from build123d import *

# Parameters (mm, degrees)
F1_DEPTH = 2.54
F3_DEPTH = 22.86
F5_DEPTH = 38.1
F6_R     = 1.5875
F7_DEPTH = 254


with BuildPart() as f1:
    # F0 (on Top) → F1 (new body)
    with BuildSketch(Plane.XY):
        with BuildLine():
            Line((-152.4, 0), (0, 0))
            Line((0, 0), (0, 85.725))
            ThreePointArc((0, 85.725), (-76.2, 9.525), (-152.4, 85.725))
            Line((-152.4, 85.725), (-152.4, 0))
        make_face()
        with BuildLine():
            ThreePointArc((-152.4, 85.725), (-76.2, 9.525), (0, 85.725))
            Line((0, 85.725), (-152.4, 85.725))
        make_face()
        with BuildLine():
            Line((-152.4, 85.725), (0, 85.725))
            ThreePointArc((0, 85.725), (-76.2, 161.925), (-152.4, 85.725))
        make_face()
    extrude(amount=F1_DEPTH)

    # F2 (on face) → F3 (join)
    with BuildSketch(Plane.XY.offset(2.54)):
        with BuildLine():
            Line((-152.4, 85.725), (0, 85.725))
            ThreePointArc((0, 85.725), (-76.2, 161.925), (-152.4, 85.725))
        make_face()
    extrude(amount=F3_DEPTH)

    # F4 (on face) → F5 (join)
    with BuildSketch(Plane.XY.offset(2.54)):
        Polygon((-3.81, 3.81), (-148.59, 3.81), (-148.59, 85.725), (-152.4, 85.725), (-152.4, 0), (0, 0), (0, 85.725), (-3.81, 85.725), align=None)
    extrude(amount=F5_DEPTH)

    # F6 (on face) → F7 (cut, symmetric)
    with BuildSketch(Plane(origin=(-152.4, 0, 0), x_dir=(0, -1, 0), z_dir=(-1, 0, 0))):
        with Locations((-68.1915506721, 18.3263123035)):
            Circle(F6_R)
    extrude(amount=F7_DEPTH, both=True, mode=Mode.SUBTRACT)


solid = f1.part
Here's how the part is built. I have some questions about the finished solid (model axes, mm). A direction names the side the tool comes from. Give positions to 0.01 mm unless a question says otherwise; leave off trailing zeros. Order: outer loops, then holes, each group sorted by start corner. A loop starts at its lowest first (then second) coordinate and runs counter-clockwise, first axis right, second up. Notation, with made-up numbers: (38, 82) -> (52, 82) arc R5 cw to (52, 89) -> close; hole circle Ø2 at (-25.75, 62). An arc over 180 degrees is marked (long way). Use a Markdown table: item, result. Add a question column.
Item 1: Imagine slicing it at B-B on z = 12.5. Please give me the cut outline in (x, y) (3 decimals), plus the area to 3 significant figures.
Item 2: Will these pins go through, and if not, where does the flat tip stop? pin 1 (23 mm diameter, centred on x = -104, y = 107, fed in from +Z); pin 2 (8 mm diameter, centred on y = 112, z = 29, fed in from -X); pin 3 (1.1 mm diameter, centred on x = -1.5, z = 32.5, fed in from +Y) (3 decimals); pin 4 (5 mm diameter, centred on y = 51, z = 30.5, fed in from +X).
Item 3: For faces 1 (the face through (-77, 2, 40.64)), 2 (the face through (-3.81, 45, 21)), 3 (the face through (-2, 85.725, 33)), which set-ups out of +Z, -Z, +X, -X, +Y, -Y let a thin tool reach every point of the face, with its end or its side?
Item 4: If we mould it in two halves opening along Y, with no side actions, what happens to faces 4 (the face through (-77, 45, 2.54)), 5 (the face through (-75, 3.81, 21)), 6 (the face through (-152.4, 43, 20)), 7 (the face through (-150, 85.725, 33))? For each: pulls with the +Y half, pulls with the -Y half, needs draft (parallel to the pull), parting line crosses it, or undercut.
Item 5: Imagine slicing it at A-A on x = -76.2. Please give me the cut outline in (y, z) (3 decimals).
Item 6: I need wall thicknesses on line 1 (X direction, y = 46.5, z = 32.5); line 2 (Z direction, x = -78, y = 47); line 3 (Z direction, x = -134, y = 129.5). Which ranges of each line are inside material? Lowest first, please.
Item 7: Imagine slicing it at C-C on z = 34. Please give me the cut outline in (x, y) (3 decimals).
Item 8: Imagine slicing it at D-D on y = 142.5. Please give me the cut outline in (x, z).
Data:
| question | item | result |
|---|---|---|
| 1 | outline | (-152.4, 0) -> (0, 0) -> (0, 85.725) arc R76.2 ccw to (-152.4, 85.725) -> close; hole (-148.59, 3.81) -> (-3.81, 3.81) -> (-3.81, 85.725) -> (-148.59, 85.725) -> close |
| 1 | area | 10,300 mm² |
| 2 | pin 1 | stops at z = 25.4 |
| 2 | pin 2 | stops at x = -148.34 |
| 2 | pin 3 | stops at y = 85.725 |
| 2 | pin 4 | stops at x = 0 |
| 3 | face 1 | +Z, +X, -X, +Y, -Y |
| 3 | face 2 | +Z |
| 3 | face 3 | +Z, +X, -X, +Y |
| 4 | face 4 | undercut |
| 4 | face 5 | undercut |
| 4 | face 6 | needs draft |
| 4 | face 7 | pulls with the +Y half |
| 5 | outline | (0, 0) -> (161.925, 0) -> (161.925, 25.4) -> (85.725, 25.4) -> (85.725, 2.54) -> (3.81, 2.54) -> (3.81, 40.64) -> (0, 40.64) -> close |
| 6 | line 1 | x = -152.4 to -148.59, -3.81 to 0 |
| 6 | line 2 | z = 0 to 2.54 |
| 6 | line 3 | z = 0 to 25.4 |
| 7 | outline | (-152.4, 0) -> (0, 0) -> (0, 85.725) -> (-3.81, 85.725) -> (-3.81, 3.81) -> (-148.59, 3.81) -> (-148.59, 85.725) -> (-152.4, 85.725) -> close |
| 8 | outline | (-127.02, 0) -> (-25.38, 0) -> (-25.38, 25.4) -> (-127.02, 25.4) -> close |
